Check sheet for the modelled part. Datum: model origin and axes. Units: mm. Coordinates: 2 decimals unless noted, no trailing zeros. Write each loop counter-clockwise with the first axis right and the second up, starting at its lowest first coordinate (ties: lowest second). Pieces come first, ordered by that corner, then holes. Notation, with made-up numbers: (-6.5, 77.5) - (19.5, 77.5) arc R19 ccw to (19.5, 96.5) - close; hole circle Ø7 at (38.5, 10). An arc over 180 degrees is marked (long way). Use one line per item in the form item = value. Start each with the question number.
1. Cross-section at D-D on x = 80. Record the boundary of the cut face in (y, z), then the cut area to 3 significant figures.
2. Go/stop test with a flat-tipped pin: pin 1 Ø2.5 at (x, y) = (139.49, 143.47) entering from -Z. Record where the tip stops, or that it passes through.
3. Cross-section at C-C on z = 0.4. Give the number of separate pieces and of enclosed holes in the cut face, then the cut area to 3 significant figures.
4. Cross-section at B-B on y = 7.5. Record the boundary of the cut face in (x, z), then the cut area to 3 significant figures.
5. Scan lines: line 1 along Y through (x, z) = (19, 1.05); line 2 along X through (y, z) = (63.5, 0.75); line 3 along Y through (x, z) = (106.5, 0.75). Record each from-to range of solid material in increasing order.
6. Cross-section at A-A on x = 48.62. Record the boundary of the cut face in (y, z).
```python
from build123d import *

# Parameters (mm, degrees)
SKETCH_1_R          = 2.1
EXTRUDE_1_DEPTH     = 2
SKETCH_3_R          = 1
CUT_EXTRUDE_1_DEPTH = 10
M4X0_7_1_D          = 3.3
M4X0_7_1_DEPTH      = 11.5
M4X0_7_1_TIP        = 0.991420021


with BuildPart() as part:
    # ｽｹｯﾁ1 → ﾎﾞｽ - 押し出し1 (new body)
    with BuildSketch(Plane.XY):
        Polygon((0, 0), (68.24, 0), (146.992249894, 68.918108191), (146.992249894, 168.01), (0, 168.01), align=None)
        with Locations((18.62, 7.5)):
            Circle(SKETCH_1_R, mode=Mode.SUBTRACT)
        with Locations((48.62, 7.5)):
            Circle(SKETCH_1_R, mode=Mode.SUBTRACT)
        with Locations((139.492249894, 93.468108191)):
            Circle(SKETCH_1_R, mode=Mode.SUBTRACT)
        with Locations((139.492249894, 143.468108191)):
            Circle(SKETCH_1_R, mode=Mode.SUBTRACT)
        with Locations((125.249072144, 59.856479125)):
            Circle(SKETCH_1_R, mode=Mode.SUBTRACT)
        with Locations((80.097280518, 20.342991391)):
            Circle(SKETCH_1_R, mode=Mode.SUBTRACT)
    extrude(amount=EXTRUDE_1_DEPTH)

    # ｽｹｯﾁ3 → ｶｯﾄ - 押し出し1 (cut)
    with BuildSketch(Plane.XY.offset(2)):
        with Locations((25, 108.01)):
            Circle(SKETCH_3_R)
        with Locations((110, 108.01)):
            Circle(SKETCH_3_R)
    extrude(amount=-CUT_EXTRUDE_1_DEPTH, mode=Mode.SUBTRACT)

    # M4x0.7 ねじ穴1
    with Locations(Plane(origin=(25, 108.01, 2), x_dir=(1, 0, 0), z_dir=(0, 0, 1))):
        with Locations((0, 0), (85, 0)):
            Hole(M4X0_7_1_D / 2, depth=M4X0_7_1_DEPTH)
            with Locations((0, 0, -(M4X0_7_1_DEPTH + M4X0_7_1_TIP / 2))):  # 118° drill point
                Cone(0, M4X0_7_1_D / 2, M4X0_7_1_TIP, mode=Mode.SUBTRACT)


solid = part.part
```
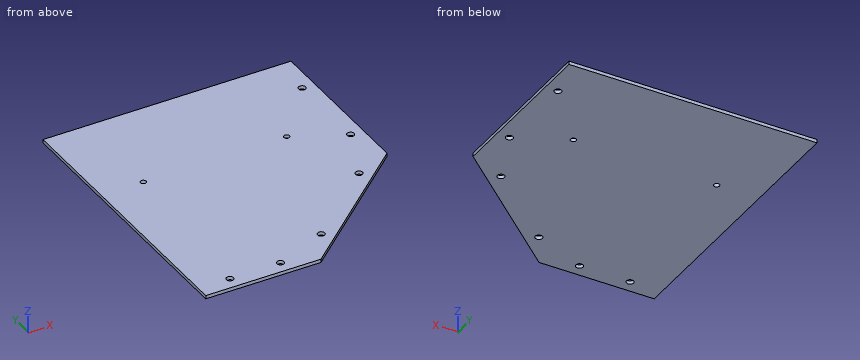
Final values:
q1.outline = (10.29, 0) - (18.25, 0) - (18.25, 2) - (10.29, 2) - close; (22.44, 0) - (168.01, 0) - (168.01, 2) - (22.44, 2) - close
q1.area = 307 mm²
q2.pin_1 = through
q3.separate_pieces = 1
q3.enclosed_holes = 8
q3.area = 21,900 mm²
q4.outline = (0, 0) - (16.52, 0) - (16.52, 2) - (0, 2) - close; (20.72, 0) - (46.52, 0) - (46.52, 2) - (20.72, 2) - close; (50.72, 0) - (76.81, 0) - (76.81, 2) - (50.72, 2) - close
q4.area = 137 mm²
q5.line_1 = 0 to 5.43, 9.57 to 168.01
q5.line_2 = 0 to 140.8
q5.line_3 = 33.48 to 168.01
q6.outline = (0, 0) - (5.4, 0) - (5.4, 2) - (0, 2) - close; (9.6, 0) - (168.01, 0) - (168.01, 2) - (9.6, 2) - close
